Design review of the part built by this model. Coordinates are the model's own, in mm. A direction names the side the tool comes from. Coordinates: 2 decimals unless noted, no trailing zeros. Loops run counter-clockwise (first coordinate to the right, second up) from the corner with the lowest first, then second, coordinate; pieces in that order, holes last.
Q1. Add section B-B on y = -11. Give the boundary of the cut face in (x, z), and give its area (3 significant figures).
Q2. Machinability: for faces 4 (the face through (10.2, -0.2, 0)), 5 (the face through (-5, 0, -2)), 6 (the face through (15.5, 0.2, -0.2)), which of the approach directions +Z, -Z, +X, -X, +Y, -Y give a long, thin tool a straight path to every point of the face, cutting with its end or side? Answer none if there is none.
Q3. Wall thickness on probe 1 along Y at (x, z) = (0, -1.35); probe 2 along Y at (x, z) = (0, -0.1); probe 3 along Y at (x, z) = (-6, -0.3): over which ranges is each line inside the solid? List them lowest first.
Q4. Draft analysis for pull direction X (two halves, no side actions). For faces 1 (the face through (-20, 0, 0)), 2 (the face through (5, 0, -2)), 3 (the face through (-27.5, -0.2, -0.9)), state which applies: released by +X, released by -X, zero draft, split by the parting line, or undercut.
Q5. Add section A-A on x = 0. Give the boundary of the cut face in (y, z).
Q6. For P1, Ø12, axis at x = 0, y = 0, coming from the +Z side; P2, Ø0.8, axis at x = 0.5, z = -2.5, coming from the +Y side; P3, Ø6, axis at x = -10, y = 9, coming from the -Z side, all flat-tipped, find the tip position at first contact; note any pin that passes through.
```python
from build123d import *

# Parameters (mm, degrees)
CUT_EXTRUDE_START    = -1.8
CUT_EXTRUDE_1_DEPTH  = 1.8
EXTRUDE_1_DEPTH      = 0.5
EXTRUDE_1_DEPTH_BACK = 2
SKETCH_3_R           = 7


with BuildPart() as part:
    # Эскиз1 → Повернуть1 (revolve)
    with BuildSketch(Plane(origin=(0, 0, 0), x_dir=(0, 0, -1), z_dir=(1, 0, 0)), mode=Mode.PRIVATE) as revolve_1_sk:
        Polygon((1.5, 7), (1.5, 8), (1, 8), (1, 9), (0.5, 9), (0.5, 10), (0, 10), (0, 15), (0.5, 15), (0.5, 15.5), (0, 15.5), (0, 27.5), (1.8, 27.5), (1.8, 7), align=None)
    revolve(revolve_1_sk.sketch.rotate(Axis((0, 0, 1.483516484), (0, 0, -1)), 90), axis=Axis((0, 0, 1.483516484), (0, 0, -1)))

    # Эскиз2 → Вырез-Вытянуть1 (cut)
    with BuildSketch(Plane.XY.offset(CUT_EXTRUDE_START)):
        with BuildLine():
            Line((-24.494897428, 12.5), (24.494897428, 12.5))
            ThreePointArc((24.494897428, 12.5), (0, 27.5), (-24.494897428, 12.5))
        make_face()
        with BuildLine():
            Line((-24.494897428, -12.5), (24.494897428, -12.5))
            ThreePointArc((24.494897428, -12.5), (0, -27.5), (-24.494897428, -12.5))
        make_face()
    extrude(amount=CUT_EXTRUDE_1_DEPTH, mode=Mode.SUBTRACT)

    # Эскиз3 → Бобышка-Вытянуть1 (add, two sides: drawn at the far end of the back side and taken through both)
    with BuildSketch(Plane.XY.offset(-1.5).offset(-EXTRUDE_1_DEPTH_BACK)):
        Circle(SKETCH_3_R)
        with BuildLine():
            Line((4, 3), (-4, 3))
            ThreePointArc((-4, 3), (-5, 0), (-4, -3))
            Line((-4, -3), (4, -3))
            ThreePointArc((4, -3), (5, 0), (4, 3))
        make_face(mode=Mode.SUBTRACT)
    extrude(amount=EXTRUDE_1_DEPTH + EXTRUDE_1_DEPTH_BACK)


solid = part.part
```
Entries:
1. outline: (-25.2, -1.8) - (25.2, -1.8) - (25.2, 0) - (10.92, 0) - (10.92, -0.5) - (10.2, -0.5) - (10.2, 0) - (-10.2, 0) - (-10.2, -0.5) - (-10.92, -0.5) - (-10.92, 0) - (-25.2, 0) - close
1. area: 90.0 mm2
2. face 4: +Z, +X, -X, +Y, -Y
2. face 5: +Z, -Z
2. face 6: +Z
3. probe 1: y = -12.5 to -8, -7 to -3, 3 to 7, 8 to 12.5
3. probe 2: y = -12.5 to -10, 10 to 12.5
3. probe 3: y = -12.5 to -8, 8 to 12.5
4. face 1: zero draft
4. face 2: undercut
4. face 3: released by -X
5. outline: (-12.5, -1.8) - (-7, -1.8) - (-7, -3.5) - (-3, -3.5) - (-3, -1) - (-7, -1) - (-7, -1.5) - (-8, -1.5) - (-8, -1) - (-9, -1) - (-9, -0.5) - (-10, -0.5) - (-10, 0) - (-12.5, 0) - close; (3, -3.5) - (7, -3.5) - (7, -1.8) - (12.5, -1.8) - (12.5, 0) - (10, 0) - (10, -0.5) - (9, -0.5) - (9, -1) - (8, -1) - (8, -1.5) - (7, -1.5) - (7, -1) - (3, -1) - close
6. P1: stops at z = -1
6. P2: stops at y = 7
6. P3: stops at z = -1.8
